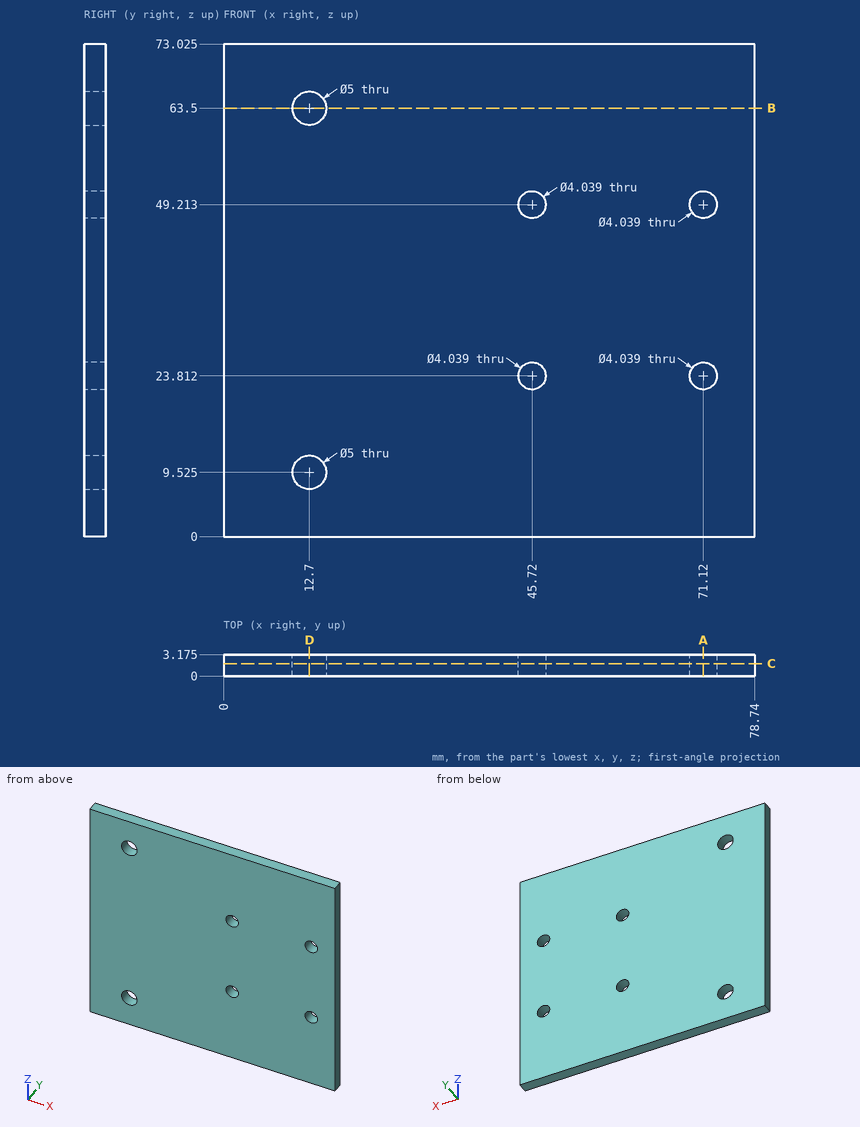
Input: dimensioned drawing with shaded views. Units: mm. Origin: part minimum x, y, z. Round coordinates to 2 decimals unless told otherwise and drop trailing zeros. Loops run counter-clockwise (first coordinate to the right, second up) from the corner with the lowest first, then second, coordinate; pieces in that order, holes last. Notation, with made-up numbers: (-18, 24) -> (23, 24) arc R20 cw to (23, 59) -> close; hole circle Ø10 at (89.25, 77). An arc over 180 degrees is marked (long way). One line per item, written item: value.
(1) Section D-D (x = 12.7). Return the cut outline in (y, z) (1 decimal).
Geometry check:
outline: (0, 0) -> (3.2, 0) -> (3.2, 7) -> (0, 7) -> close; (0, 12) -> (3.2, 12) -> (3.2, 61) -> (0, 61) -> close; (0, 66) -> (3.2, 66) -> (3.2, 73) -> (0, 73) -> close
(2) Section A-A (x = 71.12). Return the cut outline in (y, z) (1 decimal).
Geometry check:
outline: (0, 0) -> (3.2, 0) -> (3.2, 21.8) -> (0, 21.8) -> close; (0, 25.8) -> (3.2, 25.8) -> (3.2, 47.2) -> (0, 47.2) -> close; (0, 51.2) -> (3.2, 51.2) -> (3.2, 73) -> (0, 73) -> close
(3) Section B-B (z = 63.5). Return the cut outline in (x, y) (1 decimal), plus the area to 3 significant figures.
Geometry check:
outline: (0, 0) -> (10.2, 0) -> (10.2, 3.2) -> (0, 3.2) -> close; (15.2, 0) -> (78.7, 0) -> (78.7, 3.2) -> (15.2, 3.2) -> close
area: 234 mm2
(4) Section C-C (y = 1.85). Return the cut outline in (x, z) (1 decimal).
Geometry check:
outline: (0, 0) -> (78.7, 0) -> (78.7, 73) -> (0, 73) -> close; hole circle Ø5 at (12.7, 9.5); hole circle Ø5 at (12.7, 63.5); hole circle Ø4 at (45.7, 23.8); hole circle Ø4 at (45.7, 49.2); hole circle Ø4 at (71.1, 23.8); hole circle Ø4 at (71.1, 49.2)
(5) Material intervals for line 1 (Z direction, x = 12.7, y = 1.7) (1 decimal); line 2 (Z direction, x = 45.72, y = 2.3) (1 decimal); line 3 (X direction, y = 0.45, z = 22) (1 decimal), sorted ascending. Write a range as [from, to].
Geometry check:
line 1: [0, 7], [12, 61], [66, 73]
line 2: [0, 21.8], [25.8, 47.2], [51.2, 73]
line 3: [0, 44.8], [46.6, 70.2], [72, 78.7]
